Check sheet for the modelled part. Datum: model origin and axes. Units: mm. Face numbers are marked on the shaded views. A direction names the side the tool comes from. Round coordinates to 2 decimals unless told otherwise and drop trailing zeros. Write each loop counter-clockwise with the first axis right and the second up, starting at its lowest first coordinate (ties: lowest second). Pieces come first, ordered by that corner, then holes. Notation, with made-up numbers: M -7,32 L 34,32 A18 cw 34,67 Z; hole C -35.5,50 d3. An arc over 180 degrees is marked long. Answer in a Markdown table with one row per item.
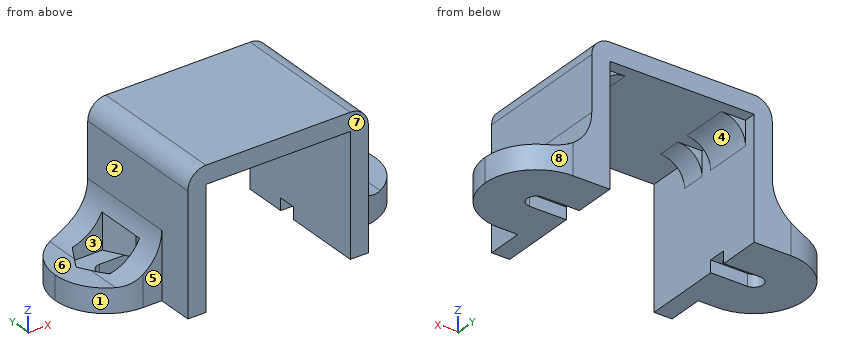
Autodesk Inventor part; units mm, degrees
ref_plane "Płaszczyzna konstrukcyjna1" through (0, 0, 1) normal (0, 0, -1) x (-1, 0, 0)
ref_plane "YZ Plane" through (0, 0, 0) normal (1, 0, 0) x (0, 1, 0)
ref_plane "XZ Plane" through (0, 0, 0) normal (0, 1, 0) x (-1, 0, 0)
sketch "Szkic1" plane through (0, 0, 0) normal (0, 0, 1) x (1, 0, 0)
  line L0 (-7.5, 5.75) -> (7.5, 5.75)
  line L1 (7.5, 5.75) -> (7.5, -5.75)
  line L2 (7.5, -5.75) -> (-7.5, -5.75)
  line L3 (-7.5, -5.75) -> (-7.5, 5.75)
  point P0 (0, 0)
  point P1 (0, 5.75)
  point P2 (-7.5, 0)
  dimension "d0" = 15
  dimension "d1" = 11.5
extrude "Wyciągnięcie proste1" add sketch "Szkic1" along normal blind 11.5
sketch "Szkic2" plane through (0, 0, 0) normal (0, 0, -1) x (-1, 0, 0)
  line L0 (7.5, 5.75) -> (-7.5, 5.75)
  line L1 (-7.5, 5.75) -> (-7.5, -5.75)
  line L2 (7.5, -5.75) -> (7.5, 5.75)
  line L3 (-13.3, 5.75) -> (13.3, 5.75)
  line L4 (13.3, 5.75) -> (13.3, -2.75)
  line L5 (13.3, -2.75) -> (-13.3, -2.75)
  line L6 (-13.3, -2.75) -> (-13.3, 5.75)
  point P0 (0, 0)
  dimension "d4" = 8.5
  dimension "d5" = 5.8
  dimension "d6" = 5.8
extrude "Wyciągnięcie proste2" add sketch "Szkic2" against normal blind 2
fillet "Zaokrąglenie1" radius 4.25 4 edges at (-13.3, -2.75, 1) (-13.3, 5.75, 1) (13.3, -2.75, 1) (13.3, 5.75, 1)
fillet "Zaokrąglenie2" radius 1.5 2 edges at (-7.5, 0, 11.5) (7.5, 0, 11.5)
fillet "Zaokrąglenie3" radius 3.5 2 edges at (-7.5, 1.5, 2) (7.5, 1.5, 2)
ref_plane "Płaszczyzna konstrukcyjna1" through (0, 0, 1) normal (0, 0, -1) x (-1, 0, 0)
sketch "Szkic3" plane through (0, 0, 1) normal (0, 0, -1) x (-1, 0, 0)
  arc A0 (-9.05, 5.75) -> (-9.05, -2.75) centre (-9.05, 1.5) ccw
  arc A1 (9.05, -2.75) -> (9.05, 5.75) centre (9.05, 1.5) ccw
  line L0 (-6.55, 1.5) -> (-7.8, -0.6651)
  line L1 (-7.8, -0.6651) -> (-10.3, -0.6651)
  line L2 (-10.3, -0.6651) -> (-11.55, 1.5)
  line L3 (-11.55, 1.5) -> (-10.3, 3.6651)
  line L4 (-10.3, 3.6651) -> (-7.8, 3.6651)
  line L5 (-7.8, 3.6651) -> (-6.55, 1.5)
  line L6 (6.55, 1.5) -> (7.8, 3.6651)
  line L7 (7.8, 3.6651) -> (10.3, 3.6651)
  line L8 (10.3, 3.6651) -> (11.55, 1.5)
  line L9 (11.55, 1.5) -> (10.3, -0.6651)
  line L10 (10.3, -0.6651) -> (7.8, -0.6651)
  line L11 (7.8, -0.6651) -> (6.55, 1.5)
  point P0 (0, 0)
  dimension "d13" = 2.5
  dimension "d14" = 18.1
extrude "Wyciągnięcie proste3" cut sketch "Szkic3" against normal blind 3
sketch "Szkic4" plane through (0, 0, 0) normal (0, 0, -1) x (-1, 0, 0)
  arc A0 (-9.05, 5.75) -> (-9.05, -2.75) centre (-9.05, 1.5) ccw
  arc A1 (9.05, -2.75) -> (9.05, 5.75) centre (9.05, 1.5) ccw
  circle A2 centre (-9.05, 1.5) radius 0.75
  circle A3 centre (9.05, 1.5) radius 0.75
  line L0 (-9.05, 2.25) -> (9.05, 2.25)
  line L1 (9.05, 0.75) -> (-9.05, 0.75)
  point P0 (0, 0)
  dimension "d17" = 1.5
extrude "Wyciągnięcie proste4" cut sketch "Szkic4" against normal blind 1
sketch "Szkic5" plane through (0, 0, 0) normal (0, 0, -1) x (-1, 0, 0)
  line L0 (-7.5, -5.75) -> (7.5, -5.75)
  line L1 (9.05, 5.75) -> (-9.05, 5.75)
  line L2 (-6, -5.75) -> (6, -5.75)
  line L3 (6, -5.75) -> (6, 5.75)
  line L4 (6, 5.75) -> (-6, 5.75)
  line L5 (-6, 5.75) -> (-6, -5.75)
  point P0 (0, 0)
  point P1 (0, 5.75)
  dimension "d20" = 12
extrude "Wyciągnięcie proste5" cut sketch "Szkic5" against normal blind 10
fillet "Zaokrąglenie4" radius 2 2 edges at (6, 0, 10) (-6, 0, 10)
sketch "Szkic7" plane through (0, 0, 0) normal (0, 0, -1) x (-1, 0, 0)
  line L0 (6, 5.75) -> (6, 2.25)
  line L1 (6, 0.75) -> (6, -5.75)
  line L2 (-6, 0.75) -> (-6, 2.25)
  line L3 (-6, 2.25) -> (-6, 5.75)
  line L4 (-6, -5.75) -> (-6, 0.75)
  line L5 (6, 2.25) -> (6, 0.75)
  line L6 (-6, 5.75) -> (6, 5.75)
  line L7 (6, 5.75) -> (6, 4.75)
  line L8 (6, 4.75) -> (-6, 4.75)
  line L9 (-6, 4.75) -> (-6, 5.75)
  line L10 (-6, 0.75) -> (6, 0.75)
  line L11 (6, 0.75) -> (6, -0.25)
  line L12 (6, -0.25) -> (-6, -0.25)
  line L13 (-6, -0.25) -> (-6, 0.75)
  line L14 (-6, -5.75) -> (6, -5.75)
  line L15 (6, -5.75) -> (6, -2.25)
  line L16 (6, -2.25) -> (-6, -2.25)
  line L17 (-6, -2.25) -> (-6, -5.75)
  point P0 (0, 0)
  dimension "d29" = 1
  dimension "d30" = 1
  dimension "d31" = 4
  dimension "d32" = 2
extrude "Wyciągnięcie proste7" cut sketch "Szkic7" against normal blind 10 contours L0 L8 L3 L6 | L1 L12 L4 L10 | L1 L14 L4 L16
equation "\"d6\" = d5"
properties part number "Mounting_bracket" material "ABS Plastic"
1. Section check B-B, the plane y = -4. Record the cut outline in (x, z), and give its area (3 significant figures).
Found:
| item | result |
|---|---|
| outline | M -7.5,0 L -6,0 L -6,10 L 6,10 L 6,0 L 7.5,0 L 7.5,10 A1.5 ccw 6,11.5 L -6,11.5 A1.5 ccw -7.5,10 Z |
| area | 51.5 mm2 |
2. Section check D-D, the plane z = 9.25. Record the cut outline in (x, y).
Found:
| item | result |
|---|---|
| outline | M -7.5,-5.75 L -6,-5.75 L -6,-2.25 L -5.56,-2.25 L -5.56,-0.25 L -6,-0.25 L -6,0.75 L -5.56,0.75 L -5.56,4.75 L -6,4.75 L -6,5.75 L -7.5,5.75 Z; M 5.56,-2.25 L 6,-2.25 L 6,-5.75 L 7.5,-5.75 L 7.5,5.75 L 6,5.75 L 6,4.75 L 5.56,4.75 L 5.56,0.75 L 6,0.75 L 6,-0.25 L 5.56,-0.25 Z |
3. Access from +Z, -Z, +X, -X, +Y, -Y to the whole of each face (thin tool, end or side, straight path). Record for the marked faces 4, 5, 6, 7 and 8.
Found:
| item | result |
|---|---|
| face 4 | -Z, +Y, -Y |
| face 5 | +Z, -Z, -X, -Y |
| face 6 | +Z, -X, +Y, -Y |
| face 7 | +Z, -Z, +X, -X, -Y |
| face 8 | +Z, -Z, +X, +Y |
4. Section check C-C, the plane x = 0.75. Record the cut outline in (y, z), and give its area (4 significant figures).
Found:
| item | result |
|---|---|
| outline | M -5.75,10 L 5.75,10 L 5.75,11.5 L -5.75,11.5 Z |
| area | 17.25 mm2 |
5. Go/stop test with flat-tipped pins: pin 1 (5 mm diameter, centred on x = 9, y = 0.5, fed in from +Z); pin 2 (2.5 mm diameter, centred on x = 12, y = 0, fed in from +Z); pin 3 (1.6 mm diameter, centred on x = -4.5, z = 9, fed in from +Y); pin 4 (1 mm diameter, centred on y = -4, z = 8.5, fed in from -X). Record where each tip stops, or that it passes through.
Found:
| item | result |
|---|---|
| pin 1 | stops at z = 11.41 |
| pin 2 | stops at z = 2.01 |
| pin 3 | passes through |
| pin 4 | stops at x = -7.5 |
6. Section check A-A, the plane z = 6.5. Record the cut outline in (x, y), and give its area (3 significant figures).
Found:
| item | result |
|---|---|
| outline | M -7.5,-5.75 L -6,-5.75 L -6,5.75 L -7.5,5.75 Z; M 6,-5.75 L 7.5,-5.75 L 7.5,5.75 L 6,5.75 Z |
| area | 34.5 mm2 |
7. Scan lines: L1, parallel to Y at x = 9.25, z = 2.25; L2, parallel to X at y = -4, z = 8.25; L3, parallel to X at y = -1, z = 3. Record each from-to range of solid material in increasing order.
Found:
| item | result |
|---|---|
| L1 | y = -2.75 to -0.67, 3.67 to 5.75 |
| L2 | x = -7.5 to -6, 6 to 7.5 |
| L3 | x = -8.55 to -6, 6 to 8.55 |
8. Draft check along Y on the marked faces 1, 2 and 3. Enter one of: +Y half, -Y half, draft (parallel to the pull), parting line (faces both ways), or undercut.
Found:
| item | result |
|---|---|
| face 1 | -Y half |
| face 2 | draft |
| face 3 | undercut |
